Build history of the part. All positions in model axes, mm. A direction names the side the tool comes from. Round coordinates to 2 decimals unless told otherwise and drop trailing zeros. Order: outer loops, then holes, each group sorted by start corner. A loop starts at its lowest first (then second) coordinate and runs counter-clockwise, first axis right, second up. Notation, with made-up numbers: M 21.5,-40 L 77.5,-40 A25 ccw 77.5,-28 Z; hole C 23.25,83 d3. An arc over 180 degrees is marked long. Use CSV: the item, a comma, the result in double quotes.
from build123d import *

# Parameters (mm, degrees)
SKETCH1_W           = 20
SKETCH1_H           = 72
BOSS_EXTRUDE1_DEPTH = 60
SKETCH2_R           = 7
CUT_EXTRUDE1_DEPTH  = 45
SKETCH3_R           = 11
CUT_EXTRUDE2_DEPTH  = 7
SKETCH4_R           = 11
CUT_EXTRUDE3_DEPTH  = 7
SKETCH5_R           = 2.65
CUT_EXTRUDE4_DEPTH  = 41
SKETCH6_R           = 5
CUT_EXTRUDE5_DEPTH  = 4
FILLET1_R           = 12
SKETCH7_R           = 5
CUT_EXTRUDE6_DEPTH  = 4


with BuildPart() as part:
    # Sketch1 → Boss-Extrude1 (new body)
    with BuildSketch(Plane.XY):
        Polygon((10, 36), (10, 56), (14, 56), (22, 19), (22, -19), (14, -56), (10, -56), (10, -36), align=None)
        Rectangle(SKETCH1_W, SKETCH1_H)
        Polygon((-14, -56), (-10, -56), (-10, -36), (-10, 36), (-10, 56), (-14, 56), (-22, 17.5), (-22, -17.5), align=None)
        Polygon((14, 56), (22, 19), (22, -19), (14, -56), align=None)
    extrude(amount=BOSS_EXTRUDE1_DEPTH)

    # Sketch2 → Cut-Extrude1 (cut, through all)
    with BuildSketch(Plane.ZY.offset(22)):
        with Locations((30, 0)):
            Circle(SKETCH2_R)
    extrude(amount=-CUT_EXTRUDE1_DEPTH, mode=Mode.SUBTRACT)

    # Sketch3 → Cut-Extrude2 (cut)
    with BuildSketch(Plane.ZY.offset(22)):
        with Locations((30, 0)):
            Circle(SKETCH3_R)
    extrude(amount=-CUT_EXTRUDE2_DEPTH, mode=Mode.SUBTRACT)

    # Sketch4 → Cut-Extrude3 (cut)
    with BuildSketch(Plane(origin=(22, 0, 0), x_dir=(0, 0, -1), z_dir=(1, 0, 0))):
        with Locations((-30, 0)):
            Circle(SKETCH4_R)
    extrude(amount=-CUT_EXTRUDE3_DEPTH, mode=Mode.SUBTRACT)

    # Sketch5 → Cut-Extrude4 (cut, through all)
    with BuildSketch(Plane(origin=(-18, 0, 0), x_dir=(0, 0, -1), z_dir=(1, 0, 0))):
        with Locations((-12, 46)):
            Circle(SKETCH5_R)
        with Locations((-48, 46)):
            Circle(SKETCH5_R)
    cut_extrude4 = extrude(amount=CUT_EXTRUDE4_DEPTH, mode=Mode.SUBTRACT)

    # Sketch6 → Cut-Extrude5 (cut)
    with BuildSketch(Plane(origin=(-18, 0, 0), x_dir=(0, 0, -1), z_dir=(1, 0, 0))):
        with Locations((-12, 46)):
            Circle(SKETCH6_R)
        with Locations((-48, 46)):
            Circle(SKETCH6_R)
    cut_extrude5 = extrude(amount=CUT_EXTRUDE5_DEPTH, mode=Mode.SUBTRACT)

    # Mirror3: Cut-Extrude4, Cut-Extrude5 across plane
    add(cut_extrude4.mirror(Plane.ZX), mode=Mode.SUBTRACT)
    add(cut_extrude5.mirror(Plane.ZX), mode=Mode.SUBTRACT)

    # Fillet1
    fillet1_edges = [part.edges().sort_by_distance(p)[0] for p in [
        (-22, -17.5, 30),
        (-22, 17.5, 30),
        (22, 19, 30),
        (22, -19, 30),
    ]]
    fillet(fillet1_edges, radius=FILLET1_R)

    # Sketch7 → Cut-Extrude6 (cut)
    with BuildSketch(Plane.ZY.offset(-18)):
        with Locations((12, 46)):
            Circle(SKETCH7_R)
        with Locations((48, 46)):
            Circle(SKETCH7_R)
    cut_extrude6 = extrude(amount=CUT_EXTRUDE6_DEPTH, mode=Mode.SUBTRACT)

    # Mirror5: Cut-Extrude6 across plane
    add(cut_extrude6.mirror(Plane.ZX), mode=Mode.SUBTRACT)


solid = part.part
(1) Cut at D-D, the plane x = 1. Give the cut face in (y, z).
Answer block:
outline,"M -36,0 L 36,0 L 36,60 L -36,60 Z; hole C 0,30 d14"
(2) Wall check: line 1 (Z direction, x = 16.05, y = -46); line 2 (Z direction, x = 11.9, y = 46); line 3 (Y direction, x = -12.65, z = 12). Give the ranges that are in metal, low to high. Write a range as from..to.
Answer block:
line 1,"z = 0..7, 17..43, 53..60"
line 2,"z = 0..9.35, 14.65..45.35, 50.65..60"
line 3,"y = -56..-48.65, -43.35..43.35, 48.65..56"
(3) Drop flat-ended pins along their axis: pin 1 (4 mm diameter, centred on y = -19.5, z = 30.5, fed in from -X); pin 2 (9 mm diameter, centred on y = -46, z = 48, fed in from +X); pin 3 (3 mm diameter, centred on y = 46, z = 48, fed in from +X); pin 4 (1.5 mm diameter, centred on x = -8.5, z = 21, fed in from +Y). Give the stop position or say it passes through.
Answer block:
pin 1,"stops at x = -21.94"
pin 2,"stops at x = 14"
pin 3,"passes through"
pin 4,"stops at y = 36"
(4) Cut at B-B, the plane y = 0. Give the cut face in (x, z), and give its area (3 significant figures).
Answer block:
outline,"M -22,0 L 22,0 L 22,19 L 15,19 L 15,23 L -15,23 L -15,19 L -22,19 Z; M -22,41 L -15,41 L -15,37 L 15,37 L 15,41 L 22,41 L 22,60 L -22,60 Z"
area,"1,910 mm²"
(5) Cut at C-C, the plane x = -12. Give the cut face in (y, z).
Answer block:
outline,"M -56,0 L 56,0 L 56,60 L -56,60 Z; hole C -46,12 d5.3; hole C -46,48 d5.3; hole C 0,30 d14; hole C 46,12 d5.3; hole C 46,48 d5.3"
(6) Tool access for faces 4 (the face through (-12, -56, 30)), 5 (the face through (0, -36, 30)), 6 (the face through (-14, 44, 10)), 7 (the face through (18.55, -10.74, 32.38)), 8 (the face through (10, 46, 30)): list every direction of +Z, -Z, +X, -X, +Y, -Y with a clear straight run to the whole face (end or side of a thin tool).
Answer block:
face 4,"+Z, -Z, +X, -X, -Y"
face 5,"+Z, -Z, -Y"
face 6,"-X"
face 7,"+X"
face 8,"+Z, -Z, +Y"
(7) Two-plate mould, pull along Z, no slides. Class faces 1 (the face through (-12.03, 48.63, 12.34)), 2 (the face through (21.93, 19.01, 30.42)), 3 (the face through (0, 1, 60)): released by +Z, released by -Z, zero draft, split by the parting line, or undercut.
Answer block:
face 1,"undercut"
face 2,"zero draft"
face 3,"released by +Z"
